The listing builds one solid part. Answer for the finished solid, in the listing's coordinates (mm). A direction names the side the tool comes from. Round coordinates to 2 decimals unless told otherwise and drop trailing zeros. Write each loop counter-clockwise with the first axis right and the second up, starting at its lowest first coordinate (ties: lowest second). Pieces come first, ordered by that corner, then holes. Notation, with made-up numbers: M -31,-0.5 L 10,-0.5 A16 ccw 10,30.5 Z; hole C 58.5,65 d8. An arc over 180 degrees is marked long. One line per item, written item: value. Start each with the question number.
(1) Section D-D (y = 32) is taken. Determine the outline of the cut face in (x, z).
(2) For a pull along X with two mould halves and no side action, classify faces 6 (the flat face through (-75, 1, 1)), 7 (the flat face through (-43.4, 0, 72)), 8 (the flat face through (-34, 1, 70)), 9 (the flat face through (24, -1, -68)) as released by +X, released by -X, zero draft, split by the parting line, or undercut.
(3) Given P1, Ø5, axis at x = 2.5, y = -25, coming from the +Z side; P2, Ø2.5, axis at y = -3.5, z = 73, coming from the -X side; P3, Ø1.5, axis at y = 10, z = 73.5, coming from the +X side; P4, Ø5.5, axis at x = -56, z = 72.5, coming from the -Y side, each flat-ended and moving along its own axis, determine where each tip first touches the part or whether it passes through.
(4) Consider probe 1 along Z at (x, y) = (-16, 35); probe 2 along Z at (x, y) = (-31, 24). Determine where each line is inside the solid, lowest interval first.
(5) Section C-C (x = -62.5) is taken. Determine the outline of the cut face in (y, z), plus the area to 3 significant figures.
(6) Section B-B (y = -6) is taken. Determine the outline of the cut face in (x, z).
(7) Section A-A (x = -36.5) is taken. Determine the outline of the cut face in (y, z).
(8) For faces 1 (the flat face through (23, -39, 68)), 2 (the flat face through (-17, 1, -65)), 3 (the flat face through (-55, -25, 72)), 4 (the flat face through (32, 1, -70)), 5 (the flat face through (-65.7, 0, 72)), determine the directions among +Z, -Z, +X, -X, +Y, -Y from which every point of the face is accessible in a straight line to the end or side of a thin tool.
```python
from build123d import *

# Parameters (mm, degrees)
SKETCH1_W           = 150
SKETCH1_H           = 140
BOSS_EXTRUDE1_DEPTH = 49
SKETCH2_W           = 83
SKETCH2_H           = 78
CUT_EXTRUDE1_DEPTH  = 5
SKETCH3_W           = 22.3
SKETCH3_H           = 50
BOSS_EXTRUDE2_DEPTH = 5
SKETCH4_W           = 84
SKETCH4_H           = 79
CUT_EXTRUDE2_DEPTH  = 5


with BuildPart() as part:
    # Sketch1 → Boss-Extrude1 (new, symmetric)
    with BuildSketch(Plane(origin=(0, 0, 0), x_dir=(1, 0, 0), z_dir=(0, 1, 0))):
        Rectangle(SKETCH1_W, SKETCH1_H)
    extrude(amount=BOSS_EXTRUDE1_DEPTH, both=True)

    # Sketch2 → Cut-Extrude1 (cut)
    with BuildSketch(Plane.XY.offset(70)):
        with Locations((23.5, 0)):
            Rectangle(SKETCH2_W, SKETCH2_H)
    extrude(amount=-CUT_EXTRUDE1_DEPTH, mode=Mode.SUBTRACT)

    # Sketch3 → Boss-Extrude2 (add)
    with BuildSketch(Plane.XY.offset(70)):
        with Locations((-54.55, 0)):
            Rectangle(SKETCH3_W, SKETCH3_H)
    extrude(amount=BOSS_EXTRUDE2_DEPTH)

    # Sketch4 → Cut-Extrude2 (cut)
    with BuildSketch(Plane(origin=(0, 0, -70), x_dir=(-1, 0, 0), z_dir=(0, 0, -1))):
        with Locations((18, 0)):
            Rectangle(SKETCH4_W, SKETCH4_H)
    extrude(amount=-CUT_EXTRUDE2_DEPTH, mode=Mode.SUBTRACT)


solid = part.part
```
Recorded:
1. outline: M -75,-70 L -60,-70 L -60,-65 L 24,-65 L 24,-70 L 75,-70 L 75,70 L 65,70 L 65,65 L -18,65 L -18,70 L -75,70 Z
2. face 6: released by -X
2. face 7: released by +X
2. face 8: zero draft
2. face 9: undercut
3. P1: stops at z = 65
3. P2: stops at x = -65.7
3. P3: stops at x = -43.4
3. P4: stops at y = -49
4. probe 1: z = -65 to 65
4. probe 2: z = -65 to 70
5. outline: M -49,-70 L 49,-70 L 49,70 L 25,70 L 25,75 L -25,75 L -25,70 L -49,70 Z
5. area: 14,000 mm2
6. outline: M -75,-70 L -60,-70 L -60,-65 L 24,-65 L 24,-70 L 75,-70 L 75,70 L 65,70 L 65,65 L -18,65 L -18,70 L -43.4,70 L -43.4,75 L -65.7,75 L -65.7,70 L -75,70 Z
7. outline: M -49,-70 L -39.5,-70 L -39.5,-65 L 39.5,-65 L 39.5,-70 L 49,-70 L 49,70 L -49,70 Z
8. face 1: +Z
8. face 2: -Z
8. face 3: +Z, +X, -X, -Y
8. face 4: -Z, +X, -X, +Y, -Y
8. face 5: +Z, -X, +Y, -Y
